Build history of the part. All positions in model axes, mm. Coordinates: 2 decimals unless noted, no trailing zeros. Order: outer loops, then holes, each group sorted by start corner. A loop starts at its lowest first (then second) coordinate and runs counter-clockwise, first axis right, second up. Notation, with made-up numbers: (-16, 47) - (9, 47) arc R17 ccw to (9, 80) - close; hole circle Ø2 at (64.5, 27). An arc over 180 degrees is marked (long way). Write each question's results on one line, items separated by ' | '.
from build123d import *

# Parameters (mm, degrees)
F0_W     = 76.2
F0_H     = 584.2
F1_DEPTH = 38.1
F2_SIZE  = 12.7


with BuildPart() as f1:
    # F0 (on Top) → F1 (new body)
    with BuildSketch(Plane.XY):
        Rectangle(F0_W, F0_H)
    extrude(amount=F1_DEPTH)

    # F2
    f2_edges = [f1.edges().sort_by_distance(p)[0] for p in [
        (0, -292.1, 38.1),
        (38.1, 0, 38.1),
        (-38.1, 0, 38.1),
    ]]
    chamfer(f2_edges, length=F2_SIZE)


solid = f1.part
1. Probe line 1 (Z direction, x = 35.5, y = 190.5); line 2 (Y direction, x = 3, z = 26); line 3 (X direction, y = -123, z = 26.5). List the from-to ranges inside material, lowest first.
Solved:
line 1: z = 0 to 28 | line 2: y = -291.5 to 292.1 | line 3: x = -37 to 37
2. Band-saw the part on B-B on z = 32.5. Give the cut face in (x, y).
Solved:
outline: (-31, -285) - (31, -285) - (31, 292.1) - (-31, 292.1) - close
3. Band-saw the part on A-A on y = 40. Give the cut face in (x, z), then the cut area to 3 significant figures.
Solved:
outline: (-38.1, 0) - (38.1, 0) - (38.1, 25.4) - (25.4, 38.1) - (-25.4, 38.1) - (-38.1, 25.4) - close | area: 2,740 mm2
